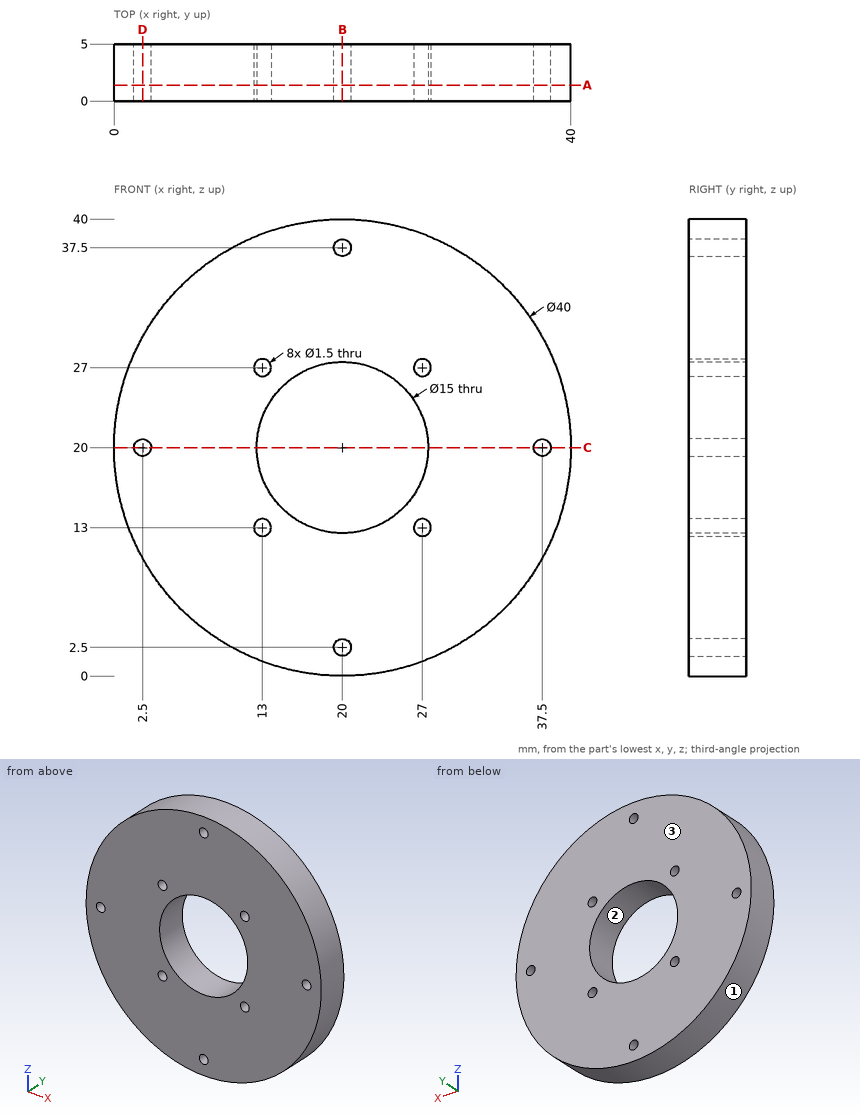
Geometry check sheet. Reference: drawing and pictorial views, mm from the part's lowest x, y, z. Coordinates: 2 decimals unless noted, no trailing zeros. Loops run counter-clockwise (first coordinate to the right, second up) from the corner with the lowest first, then second, coordinate; pieces in that order, holes last.
1) Release check for a two-part mould opening along X. For the marked faces 1, 2 and 3 record: released by +X, released by -X, zero draft, split by the parting line, or undercut.
2) Material ranges on probe 1 along X at (y, z) = (1.55, 20); probe 2 along Z at (x, y) = (37, 4.7); probe 3 along X at (y, z) = (3.6, 2.5), recorded low to high.
3) Sectioned sample at A-A (y = 1.4). Count the separate pieces of the cut face and the enclosed holes in it, and give its area (3 significant figures).
4) Gauge pin test, flat ends, axial feed: pin 1 (3 mm diameter, centred on y = 4, z = 8.5, fed in from -X); pin 2 (3 mm diameter, centred on x = 24.5, y = 2.5, fed in from -Z). Record the tip position at first contact, or that the pin passes through.
5) Sectioned sample at B-B (x = 20). Record the boundary of the cut face in (y, z), and give its area (3 significant figures).
6) Sectioned sample at D-D (x = 2.5). Record the boundary of the cut face in (y, z).
7) Sectioned sample at C-C (z = 20). Record the boundary of the cut face in (x, y).
Check sheet entries:
1. face 1: split by the parting line
1. face 2: undercut
1. face 3: zero draft
2. probe 1: x = 0 to 1.75, 3.25 to 12.5, 27.5 to 36.75, 38.25 to 40
2. probe 2: z = 9.46 to 19.44, 20.56 to 30.54
2. probe 3: x = 10.32 to 19.25, 20.75 to 29.68
3. separate pieces: 1
3. enclosed holes: 9
3. area: 1,070 mm2
4. pin 1: stops at x = 2.68
4. pin 2: stops at z = 0.23
5. outline: (0, 0) - (5, 0) - (5, 1.75) - (0, 1.75) - close; (0, 3.25) - (5, 3.25) - (5, 12.5) - (0, 12.5) - close; (0, 27.5) - (5, 27.5) - (5, 36.75) - (0, 36.75) - close; (0, 38.25) - (5, 38.25) - (5, 40) - (0, 40) - close
5. area: 110 mm2
6. outline: (0, 10.32) - (5, 10.32) - (5, 19.25) - (0, 19.25) - close; (0, 20.75) - (5, 20.75) - (5, 29.68) - (0, 29.68) - close
7. outline: (0, 0) - (1.75, 0) - (1.75, 5) - (0, 5) - close; (3.25, 0) - (12.5, 0) - (12.5, 5) - (3.25, 5) - close; (27.5, 0) - (36.75, 0) - (36.75, 5) - (27.5, 5) - close; (38.25, 0) - (40, 0) - (40, 5) - (38.25, 5) - close
